Design review of the part built by this model. Coordinates are the model's own, in mm. Give positions to 0.01 mm unless a question says otherwise; leave off trailing zeros. Loops run counter-clockwise (first coordinate to the right, second up) from the corner with the lowest first, then second, coordinate; pieces in that order, holes last. Notation, with made-up numbers: (65, -8) -> (80, -8) arc R13 cw to (80, -1) -> close; hole circle Ø6 at (16.5, 49). An arc over 180 degrees is marked (long way). Use CSV: the item, a comma, the result in double quotes. Start each with the question number.
Item 1: We need section A-A (z = -3.75). State the section outline as (x, y) points, plus the area to 3 significant figures.
Item 2: Wall thickness on line 1 along Y through (x, z) = (38.5, 1.25); line 2 along X through (y, z) = (-47.5, 11.25); line 3 along Y through (x, z) = (63, 6.75): over which ranges is each line inside the solid? List them lowest first. Write a range as from..to.
Item 3: Clearance check with flat-ended pins moving along their axes: pin 1 (1.5 mm diameter, centred on y = -23, z = 9, fed in from +X); pin 2 (1.5 mm diameter, centred on y = -68.5, z = 4, fed in from -X); pin 3 (6 mm diameter, centred on y = -91, z = -3.5, fed in from +X). State where each tip first meets the part, or that it passes through.
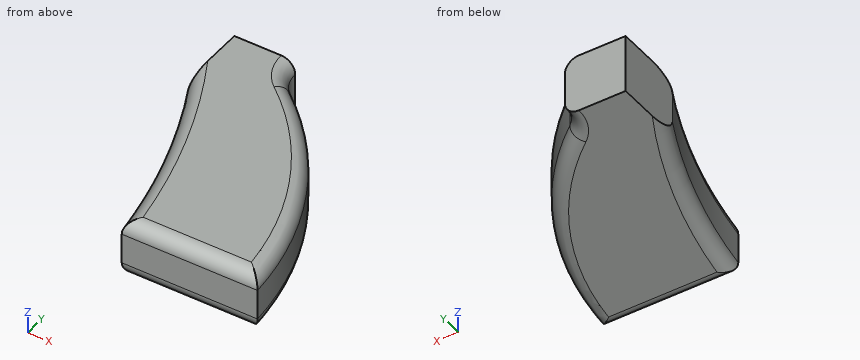
from build123d import *

# Parameters (mm, degrees)
EXTRUDE_1_DEPTH = 12.5
FILLET_1_R      = 6


with BuildPart() as part:
    # 草图1 → 凸台-拉伸1 (new, symmetric)
    with BuildSketch(Plane.XY):
        with BuildLine():
            Line((0, 0), (26, 0))
            ThreePointArc((26, 0), (27.468456661, -6.472815065), (31.586311315, -11.678290343))
            ThreePointArc((31.586311315, -11.678290343), (67.528745318, -55.48682347), (83, -110))
            Line((83, -110), (25, -110))
            ThreePointArc((25, -110), (15.68286649, -69.005354222), (0, -30))
            Line((0, -30), (0, 0))
        make_face()
    extrude(amount=EXTRUDE_1_DEPTH, both=True)

    # 圆角1
    fillet_1_edges = [part.edges().sort_by_distance(p)[0] for p in [
        (54, -110, 12.5),
        (67.528745318, -55.48682347, 12.5),
        (27.468456661, -6.472815065, 12.5),
        (27.468456661, -6.472815065, -12.5),
        (67.528745318, -55.48682347, -12.5),
        (54, -110, -12.5),
        (15.68286649, -69.005354222, -12.5),
        (15.68286649, -69.005354222, 12.5),
    ]]
    fillet(fillet_1_edges, radius=FILLET_1_R)


solid = part.part
Results found:
1,outline,"(0, -30) arc R265 cw to (25, -110) -> (83, -110) arc R139 ccw to (31.59, -11.68) arc R15 cw to (26, 0) -> (0, 0) -> close"
1,area,"5,630 mm²"
2,line 1,"-110..-17.64"
2,line 2,"10.45..60.27"
2,line 3,"-109.99..-47.49"
3,pin 1,"x = 44.1"
3,pin 2,"x = 15.29"
3,pin 3,"x = 80.92"
